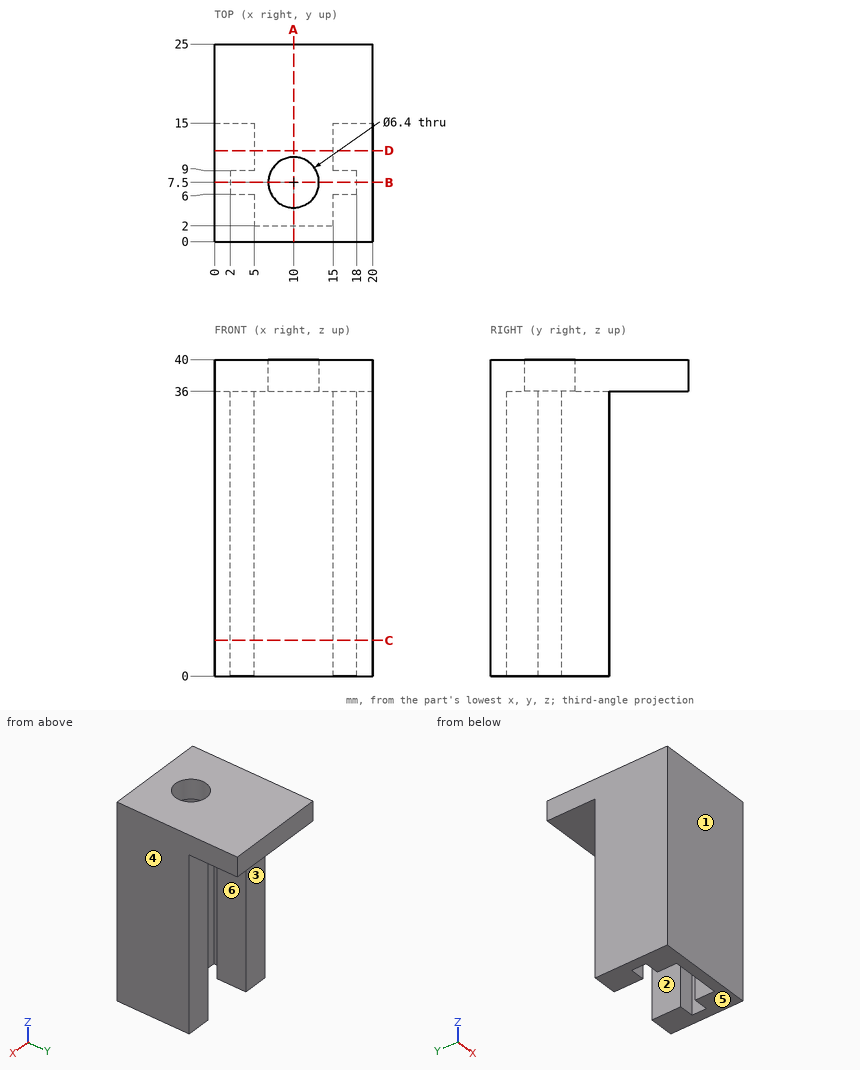
Answer from the drawing. Dimensions are ordinates in mm from the lowest x, y and z of the part. A direction names the side the tool comes from. Round coordinates to 2 decimals unless told otherwise and drop trailing zeros. Write each loop counter-clockwise with the first axis right and the second up, starting at its lowest first coordinate (ties: lowest second). Pieces come first, ordered by that corner, then holes. Notation, with made-up numbers: M 11.25,52.5 L 35.25,52.5 A33 ccw 35.25,80.5 Z; hole C 81.25,56 d11. An arc over 180 degrees is marked long. Write each question's results on one line, items separated by ' | '. Start each with the question number.
Item 1: The mould has two halves that part along X. Classify the marked faces 4, 5 and 6: +X half, -X half, draft (parallel to the pull), parting line (faces both ways), or undercut.
Item 2: Find section D-D on y = 11.5. Write down the section's boundary in (x, z), and give its area (3 significant figures).
Item 3: Find section A-A on x = 10. Write down the section's boundary in (y, z), and give its area (3 significant figures).
Item 4: Find section B-B on y = 7.5. Write down the section's boundary in (x, z).
Item 5: Given pin 1 Ø2.5 at (x, z) = (2.5, 18.5) entering from +Y; pin 2 Ø1.5 at (x, z) = (12.5, 7.5) entering from +Y; pin 3 Ø4 at (x, y) = (10, 7.5) entering from -Z, each flat-ended and moving along its own axis, determine where each tip first touches the part or whether it passes through.
Item 6: Straight lines are drawn through the part: probe 1 along Y at (x, z) = (2.25, 18); probe 2 along Y at (x, z) = (10, 38.95); probe 3 along X at (y, z) = (12, 21.5). For each, find the intervals that lie inside material, in ascending order.
Item 7: Find section C-C on z = 4.5. Write down the section's boundary in (x, y), and give its area (3 significant figures).
Item 8: Which of the six approach directions +Z, -Z, +X, -X, +Y, -Y give full straight-line access (tool end or side, diameter ignored) to the marked faces 1, 2 and 3?
Answer block:
1) face 4: +X half | face 5: draft | face 6: undercut
2) outline: M 0,0 L 5,0 L 5,36 L 15,36 L 15,0 L 20,0 L 20,40 L 0,40 Z | area: 440 mm²
3) outline: M 0,0 L 2,0 L 2,36 L 4.3,36 L 4.3,40 L 0,40 Z; M 10.7,36 L 25,36 L 25,40 L 10.7,40 Z | area: 146 mm²
4) outline: M 0,0 L 2,0 L 2,36 L 6.8,36 L 6.8,40 L 0,40 Z; M 13.2,36 L 18,36 L 18,0 L 20,0 L 20,40 L 13.2,40 Z
5) pin 1: stops at y = 15 | pin 2: stops at y = 2 | pin 3: passes through
6) probe 1: y = 0 to 6, 9 to 15 | probe 2: y = 0 to 4.3, 10.7 to 25 | probe 3: x = 0 to 5, 15 to 20
7) outline: M 0,0 L 20,0 L 20,15 L 15,15 L 15,9 L 18,9 L 18,6 L 15,6 L 15,2 L 5,2 L 5,6 L 2,6 L 2,9 L 5,9 L 5,15 L 0,15 Z | area: 152 mm²
8) face 1: +Z, -Z, +X, -X, -Y | face 2: -Z, +Y | face 3: -Z, +X, -X, +Y
